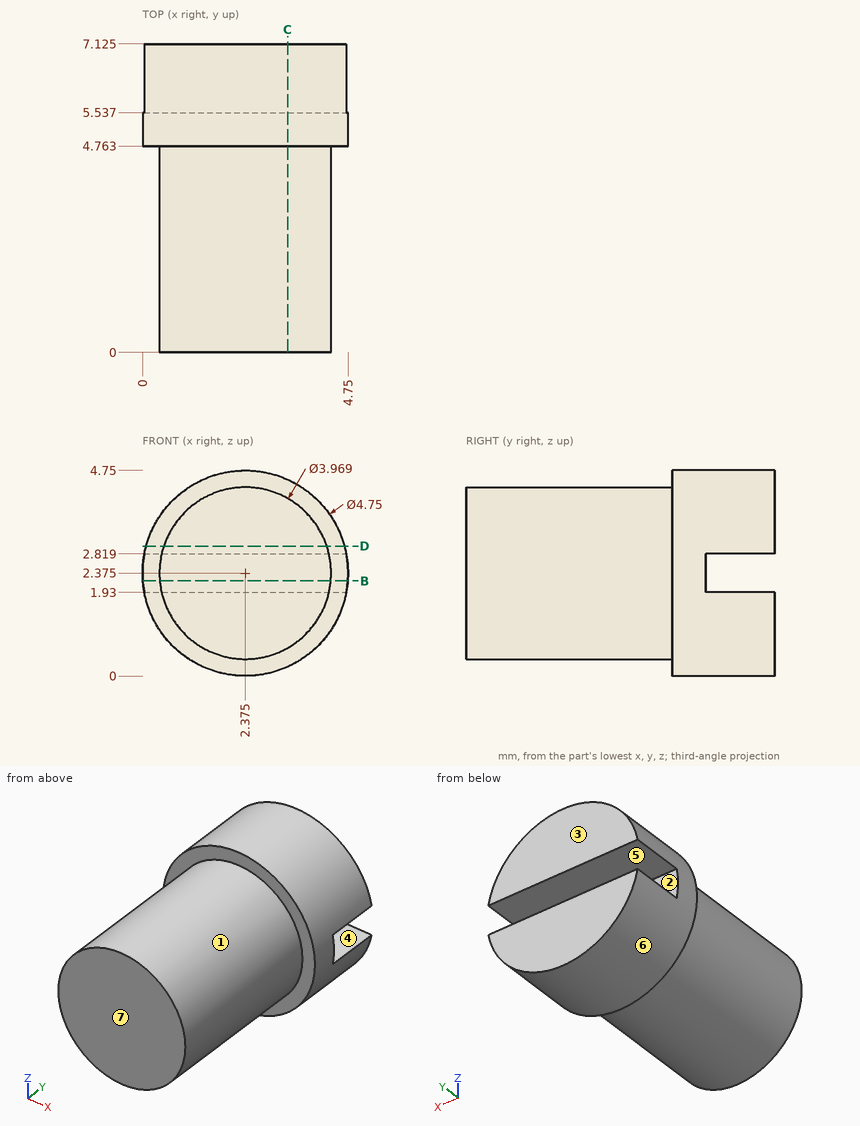
Answer from the drawing. Dimensions are ordinates in mm from the lowest x, y and z of the part. A direction names the side the tool comes from. Round coordinates to 2 decimals unless told otherwise and drop trailing zeros. Write each loop counter-clockwise with the first axis right and the second up, starting at its lowest first coordinate (ties: lowest second). Pieces come first, ordered by that corner, then holes. Notation, with made-up numbers: (23.25, 50) -> (45.25, 50) arc R22 cw to (45.25, 57) -> close; hole circle Ø4 at (17, -10). An arc over 180 degrees is marked (long way). Answer in a Markdown table with one row per item. Add a question column.
1) Find section C-C, the plane x = 3.35. Determine the outline of the cut face in (y, z) (1 decimal), and give its area (3 significant figures).
2) Find section B-B, the plane z = 2.2. Determine the outline of the cut face in (x, y).
3) Given P1, Ø1, axis at x = 3.5, y = 4, coming from the +Z side, flat-ended and moving along its own axis, determine where the tip first touches the part or whether it passes through.
4) Consider line 1 (Y direction, x = 3.6, z = 4) (1 decimal); line 2 (Y direction, x = 3.4, z = 2.2); line 3 (Z direction, x = 2.55, y = 6.75). Determine where each line is inside the solid, lowest interval first.
5) Find section D-D, the plane z = 3. Determine the outline of the cut face in (x, y) (1 decimal).
6) Which of the six approach directions +Z, -Z, +X, -X, +Y, -Y give full straight-line access (tool end or side, diameter ignored) to the marked faces 1, 2 and 3?
7) Determine the mould class of the marked faces 4, 5, 6 and 7 for opening direction Z: pulls with the +Z half, pulls with the -Z half, needs draft (parallel to the pull), parting line crosses it, or undercut.
Findings below:
| question | item | result |
|---|---|---|
| 1 | outline | (0, 0.6) -> (4.8, 0.6) -> (4.8, 0.2) -> (7.1, 0.2) -> (7.1, 1.9) -> (5.5, 1.9) -> (5.5, 2.8) -> (7.1, 2.8) -> (7.1, 4.5) -> (4.8, 4.5) -> (4.8, 4.1) -> (0, 4.1) -> close |
| 1 | area | 25.3 mm² |
| 2 | outline | (0.01, 4.76) -> (0.4, 4.76) -> (0.4, 0) -> (4.35, 0) -> (4.35, 4.76) -> (4.74, 4.76) -> (4.74, 5.54) -> (0.01, 5.54) -> close |
| 3 | P1 | z = 4.26 |
| 4 | line 1 | 4.8 to 7.1 |
| 4 | line 2 | 0 to 5.54 |
| 4 | line 3 | 0.01 to 1.93, 2.82 to 4.74 |
| 5 | outline | (0.1, 4.8) -> (0.5, 4.8) -> (0.5, 0) -> (4.3, 0) -> (4.3, 4.8) -> (4.7, 4.8) -> (4.7, 7.1) -> (0.1, 7.1) -> close |
| 6 | face 1 | -Y |
| 6 | face 2 | +X, -X, +Y |
| 6 | face 3 | +Z, -Z, +X, -X, +Y |
| 7 | face 4 | undercut |
| 7 | face 5 | undercut |
| 7 | face 6 | parting line crosses it |
| 7 | face 7 | needs draft |
